Could you check a few things on this drawing? It's one solid part, dimensions in mm from its lowest x, y, z. Coordinates: 2 decimals unless noted, no trailing zeros. Order: outer loops, then holes, each group sorted by start corner. A loop starts at its lowest first (then second) coordinate and runs counter-clockwise, first axis right, second up.
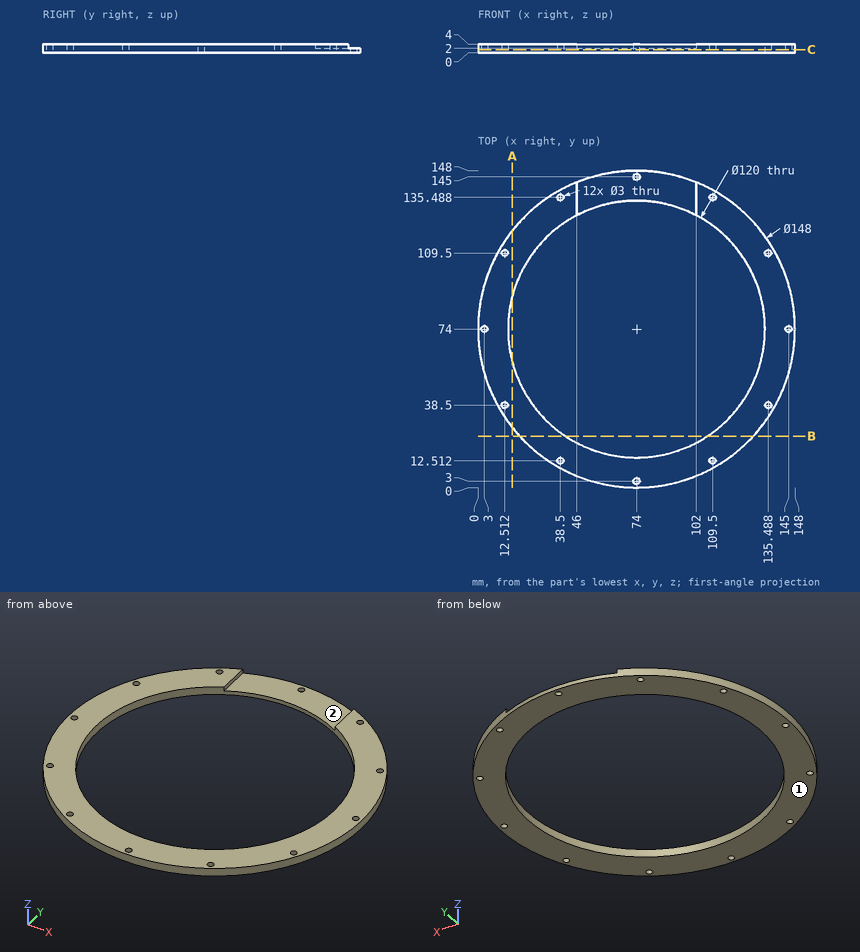
1. Thinking about a two-plate mould opening in X: for the marked faces 1 and 2, which applies, pulls with the +X half, pulls with the -X half, needs draft (parallel to the pull), parting line crosses it, or undercut?
Completed:
face 1: needs draft
face 2: undercut
2. Imagine slicing it at B-B on y = 24. Please give me the cut outline in (x, z), then the cut area to 3 significant figures.
Completed:
outline: (19.45, 0) - (40.83, 0) - (40.83, 4) - (19.45, 4) - close; (107.17, 0) - (128.55, 0) - (128.55, 4) - (107.17, 4) - close
area: 171 mm2
3. Imagine slicing it at A-A on x = 16. Please give me the cut outline in (y, z), then the cut area to 3 significant figures.
Completed:
outline: (28.04, 0) - (58.64, 0) - (58.64, 4) - (28.04, 4) - close; (89.36, 0) - (119.96, 0) - (119.96, 4) - (89.36, 4) - close
area: 245 mm2
4. Imagine slicing it at C-C on z = 1.35. Give the number of separate pieces and of enclosed holes in the cut face, then the cut area to 3 significant figures.
Completed:
separate pieces: 1
enclosed holes: 13
area: 5,810 mm2
5. I'm going to push flat-ended pins straight in: pin 1 (2 mm diameter, centred on y = 133.5, z = 3, fed in from -X); pin 2 (4 mm diameter, centred on x = 12.51, y = 38.5, fed in from -Z); pin 3 (23 mm diameter, centred on x = 72.5, y = 134.5, fed in from +Z); pin 4 (1.6 mm diameter, centred on y = 135, z = 3, fed in from +X) (1 decimal). Where does each tip first touch, or does it pass through?
Completed:
pin 1: stops at x = 28.68
pin 2: stops at z = 0
pin 3: stops at z = 2
pin 4: stops at x = 117
6. Please list where these lines run through material, in increasing order: probe 1 along X at (y, z) = (74, 2.65); probe 2 along X at (y, z) = (136, 0.35); probe 3 along X at (y, z) = (73, 2.1).
Completed:
probe 1: x = 0 to 1.5, 4.5 to 14, 134 to 143.5, 146.5 to 148
probe 2: x = 33.6 to 37.09, 39.91 to 108.09, 110.91 to 114.4
probe 3: x = 0.01 to 1.88, 4.12 to 14.01, 133.99 to 143.88, 146.12 to 147.99
